Here's the drawing with two shaded views (mm, measured from the low corner). I have some questions. Round coordinates to 2 decimals unless told otherwise and drop trailing zeros. Order: outer loops, then holes, each group sorted by start corner. A loop starts at its lowest first (then second) coordinate and runs counter-clockwise, first axis right, second up. Notation, with made-up numbers: (72, -37) -> (122, -37) arc R11 cw to (122, -30) -> close; hole circle Ø10 at (51, 70.25). An arc over 180 degrees is marked (long way). Use a Markdown table: item, result. Add a question column.
Q1. I need wall thicknesses on line 1 along X through (y, z) = (48.5, 2.65); line 2 along Y through (x, z) = (29, 2); line 3 along X through (y, z) = (56.22, 1.95). Which ranges of each line are inside material? Lowest first, please. Write a range as [from, to].
Q2. I'm going to push flat-ended pins straight in: pin 1 Ø8 at (x, y) = (111, 43) entering from -Z; pin 2 Ø3 at (x, y) = (23.5, 12.5) entering from -Z. Where does each tip first touch, or does it pass through?
Q3. If we section it at B-B on z = 1.8: Give the number of separate pieces and of enclosed holes in the cut face, plus the area to 3 significant figures.
Q4. If we section it at A-A on y = 47: List the corners of the cut face in (x, z) for me, plus the area to 3 significant figures.
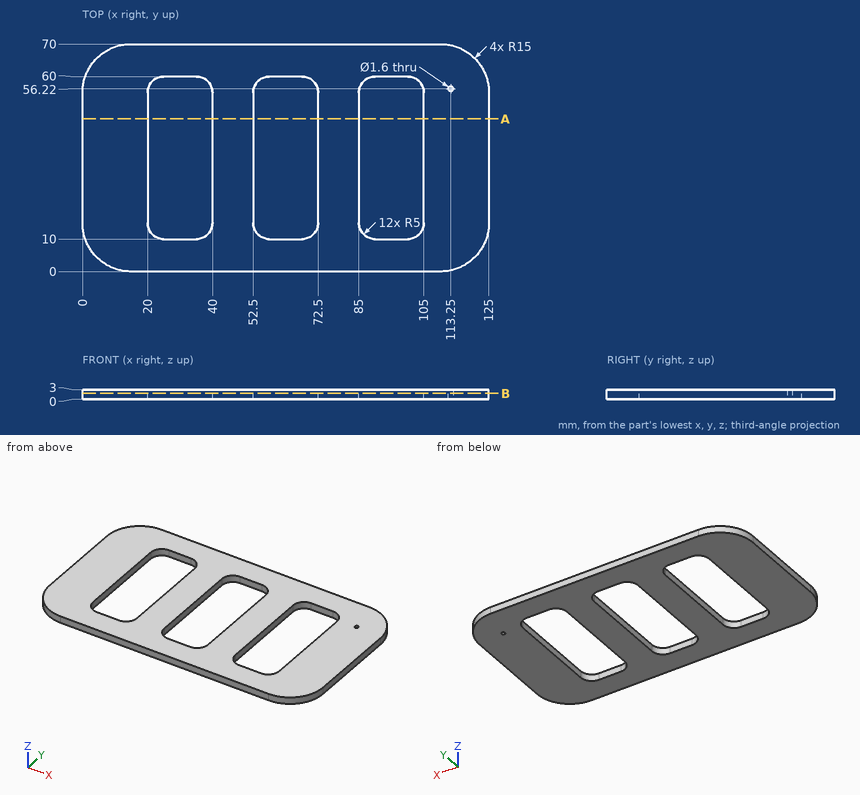
Answer below:
| question | item | result |
|---|---|---|
| 1 | line 1 | [0, 20], [40, 52.5], [72.5, 85], [105, 125] |
| 1 | line 2 | [0, 10], [60, 70] |
| 1 | line 3 | [0.05, 20.15], [39.85, 52.65], [72.35, 85.15], [104.85, 112.45], [114.05, 124.95] |
| 2 | pin 1 | z = 0 |
| 2 | pin 2 | through |
| 3 | separate pieces | 1 |
| 3 | enclosed holes | 4 |
| 3 | area | 5,620 mm² |
| 4 | outline | (0, 0) -> (20, 0) -> (20, 3) -> (0, 3) -> close; (40, 0) -> (52.5, 0) -> (52.5, 3) -> (40, 3) -> close; (72.5, 0) -> (85, 0) -> (85, 3) -> (72.5, 3) -> close; (105, 0) -> (125, 0) -> (125, 3) -> (105, 3) -> close |
| 4 | area | 195 mm² |
